Here's how the part is built. I have some questions about the finished solid (model axes, mm). Face numbers are marked on the shaded views. Give positions to 0.01 mm unless a question says otherwise; leave off trailing zeros. Write each loop counter-clockwise with the first axis right and the second up, starting at its lowest first coordinate (ties: lowest second). Pieces come first, ordered by that corner, then holes. Notation, with made-up numbers: (72.25, -23) -> (106.25, -23) arc R11 ccw to (106.25, -3) -> close; hole circle Ø4 at (-31.75, 24). An arc over 180 degrees is marked (long way). Use one line per item in the form item = value.
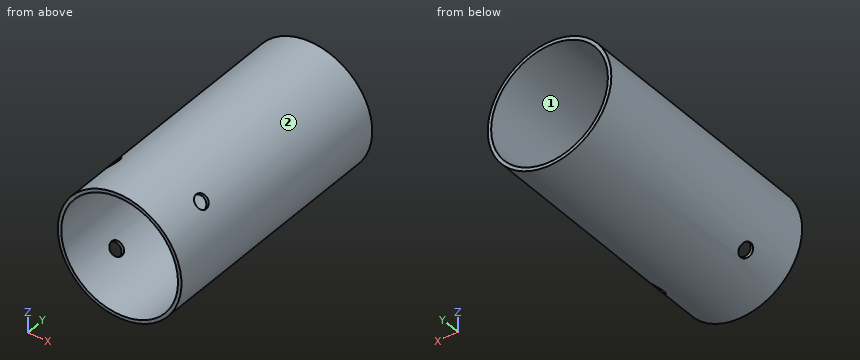
```python
from build123d import *

# Parameters (mm, degrees)
SKETCH1_W          = 0.85
SKETCH1_H          = 63.5
SKETCH2_R          = 1.778
CUT_EXTRUDE1_DEPTH = 2.54
CIRPATTERN1_COUNT  = 4


with BuildPart() as part:
    # Sketch1 → Revolve1 (revolve)
    with BuildSketch(Plane.XY):
        with Locations((-14.925, 285.75)):
            Rectangle(SKETCH1_W, SKETCH1_H)
    revolve(axis=Axis((0, 0, 0), (0, 1, 0)))

    # Sketch2 → Cut-Extrude1 (cut)
    with BuildSketch(Plane(origin=(-10.854089091, 0, 10.854089091), x_dir=(0, -1, 0), z_dir=(-0.707106781, 0, 0.707106781))):
        with Locations((-266.7, 0)):
            Circle(SKETCH2_R)
    cut_extrude1 = extrude(amount=-CUT_EXTRUDE1_DEPTH, mode=Mode.SUBTRACT)

    # CirPattern1: Cut-Extrude1 ×4 about axis
    cirpattern1_axis = Axis((0, 317.5, 0), (0, -1, 0))
    for i in range(1, CIRPATTERN1_COUNT):
        add(cut_extrude1.rotate(cirpattern1_axis, i * 360 / CIRPATTERN1_COUNT), mode=Mode.SUBTRACT)


solid = part.part
```
Q1. Will these pins go through, and if not, where does the flat tip stop? pin 1 Ø1 at (y, z) = (295, -2) entering from +X; pin 2 Ø5 at (y, z) = (266, 9.5) entering from -X; pin 3 Ø1.5 at (y, z) = (278, -9.5) entering from +X.
Result set:
pin_1 = 15.28
pin_2 = -13.66
pin_3 = 12.61
Q2. I want a section at A-A, the plane z = 0. Write out the boundary of the cut face in (x, y).
Result set:
outline = (-15.35, 254) -> (-14.5, 254) -> (-14.5, 317.5) -> (-15.35, 317.5) -> close; (14.5, 254) -> (15.35, 254) -> (15.35, 317.5) -> (14.5, 317.5) -> close
Q3. If I drill on line 1 along Z through (x, y) = (0, 272); line 2 along X through (y, z) = (271, 9); line 3 along X through (y, z) = (303, -5.5), over which ranges is the centre line in solid material (lowest first)? Write a range as from..to.
Result set:
line_1 = -15.35..-14.5, 14.5..15.35
line_2 = -12.43..-11.37, 11.37..12.43
line_3 = -14.33..-13.42, 13.42..14.33
Q4. I want a section at B-B, the plane x = 0. Write out the boundary of the cut face in (y, z), and give its area (3 significant figures).
Result set:
outline = (254, -15.35) -> (317.5, -15.35) -> (317.5, -14.5) -> (254, -14.5) -> close; (254, 14.5) -> (317.5, 14.5) -> (317.5, 15.35) -> (254, 15.35) -> close
area = 108 mm2
Q5. If we mould it in two halves opening along Z, with no side actions, what happens to the marked faces 1 and 2? For each: +Z half, -Z half, draft (parallel to the pull), parting line (faces both ways), or undercut.
Result set:
face_1 = undercut
face_2 = parting line
Q6. I want a section at C-C, the plane y = 264. Write out the boundary of the cut face in (x, z), and give its area (3 significant figures).
Result set:
outline = circle Ø30.7 at (0, 0); hole circle Ø29 at (0, 0)
area = 79.7 mm2
